from build123d import *

# Parameters (mm, degrees)
SKETCH_1_W          = 3
SKETCH_1_H          = 10
SKETCH_1_W_2        = 10
SKETCH_1_H_2        = 3
EXTRUDE_1_DEPTH     = 3
SKETCH_2_R          = 1.6
SKETCH_2_R_2        = 0.75
CUT_EXTRUDE_1_DEPTH = 57.648036153
FILLET_1_R          = 2


with BuildPart() as part:
    # 草图1 → 凸台-拉伸1 (new body)
    with BuildSketch(Plane(origin=(0, 0, 0), x_dir=(1, 0, 0), z_dir=(0, 1, 0))):
        Polygon((40, 0), (0, 0), (0, 40), align=None)
        with Locations((-1.5, 20)):
            Rectangle(SKETCH_1_W, SKETCH_1_H)
        with Locations((20, -1.5)):
            Rectangle(SKETCH_1_W_2, SKETCH_1_H_2)
    extrude(amount=EXTRUDE_1_DEPTH)

    # 草图2 → 切除-拉伸1 (cut, through all)
    with BuildSketch(Plane(origin=(0, 3, 0), x_dir=(1, 0, 0), z_dir=(0, 1, 0))):
        with Locations(Location((5, 5, 0), (0, 0, 270))):
            Circle(SKETCH_2_R)
        with Locations((0, 25)):
            Circle(SKETCH_2_R_2)
        with Locations((0, 15)):
            Circle(SKETCH_2_R_2)
        with Locations((15, 0)):
            Circle(SKETCH_2_R_2)
        with Locations((25, 0)):
            Circle(SKETCH_2_R_2)
        Polygon((5, 28.169760455), (5, 8.169760455), (25, 8.169760455), align=None)
    extrude(amount=-CUT_EXTRUDE_1_DEPTH, mode=Mode.SUBTRACT)

    # 圆角1
    fillet_1_edges = [part.edges().sort_by_distance(p)[0] for p in [
        (0, 1.5, -40),
        (40, 1.5, 0),
    ]]
    fillet(fillet_1_edges, radius=FILLET_1_R)


solid = part.part
Check sheet for the modelled part. Datum: model origin and axes. Units: mm. A direction names the side the tool comes from. Round coordinates to 2 decimals unless told otherwise and drop trailing zeros. Order: outer loops, then holes, each group sorted by start corner. A loop starts at its lowest first (then second) coordinate and runs counter-clockwise, first axis right, second up.
Q1. Draft check along Z on faces 4 (the face through (0.51, 1.52, -24.45)), 5 (the face through (20, 1, -20)), 6 (the face through (0, 1, -7)). Enter one of: pulls with the +Z half, pulls with the -Z half, needs draft (parallel to the pull), parting line crosses it, or undercut.
Filled sheet:
face 4: undercut
face 5: pulls with the -Z half
face 6: needs draft
Q2. Cross-section at C-C, the plane y = 2. Enter the section's corners in (x, z), plus the area to 3 significant figures.
Filled sheet:
outline: (-3, -25) - (-0.75, -25) arc R0.75 cw (long way) to (0, -25.75) - (0, -35.17) arc R2 ccw to (3.41, -36.59) - (36.59, -3.41) arc R2 ccw to (35.17, 0) - (25.75, 0) arc R0.75 cw (long way) to (25, 0.75) - (25, 3) - (15, 3) - (15, 0.75) arc R0.75 cw (long way) to (14.25, 0) - (0, 0) - (0, -14.25) arc R0.75 cw (long way) to (-0.75, -15) - (-3, -15) - close; hole circle Ø3.2 at (5, -5); hole (5, -28.17) - (25, -8.17) - (5, -8.17) - close
area: 637 mm2
Q3. Set-up check for faces 1 (the face through (-2, 1, -25)), 2 (the face through (31, 1, 0)), 3 (the face through (15.14, 1.52, -18.03)): record each of +Z, -Z, +X, -X, +Y, -Y from which the full face is reachable in a straight line by a thin tool's end or side.
Filled sheet:
face 1: -Z, -X, +Y, -Y
face 2: +Z, +X, +Y, -Y
face 3: +Y, -Y
Q4. Cross-section at B-B, the plane x = 8. Enter the section's corners in (y, z), plus the area to 3 significant figures.
Filled sheet:
outline: (0, -32) - (3, -32) - (3, -25.17) - (0, -25.17) - close; (0, -8.17) - (3, -8.17) - (3, 0) - (0, 0) - close
area: 45.0 mm2
Q5. Scan lines: L1, parallel to X at y = 2.8, z = -24.5; L2, parallel to Z at x = 18.5, y = 2.6; L3, parallel to X at y = 1.3, z = -18.5. Record each from-to range of solid material in increasing order.
Filled sheet:
L1: x = -3 to -0.56, 0.56 to 5, 8.67 to 15.5
L2: z = -21.5 to -14.67, -8.17 to 3
L3: x = -3 to 5, 14.67 to 21.5
Q6. Depth check by flat-ended pin: P1, Ø1.2, axis at x = 25, z = 0, coming from the -Y side; P2, Ø0.9, axis at y = 1.5, z = -32, coming from the -X side; P3, Ø1.1, axis at y = 2, z = 1.5, coming from the +X side; P4, Ø1.5, axis at x = 31, y = 1.5, coming from the +Z side. Enter the tip coordinate at first touch or a pass-through.
Filled sheet:
P1: passes through
P2: stops at x = 0
P3: stops at x = 25
P4: stops at z = 0
Q7. Cross-section at A-A, the plane z = -5. Enter the section's corners in (x, y).
Filled sheet:
outline: (0, 0) - (3.4, 0) - (3.4, 3) - (0, 3) - close; (6.6, 0) - (35, 0) - (35, 3) - (6.6, 3) - close
